```python
from build123d import *

# Parameters (mm, degrees)
SKETCH2_W               = 34
SKETCH2_H               = 40
BOSS_EXTRUDE1_DEPTH     = 3
SKETCH3_W               = 5
SKETCH3_H               = 40
BOSS_EXTRUDE2_DEPTH     = 37
CUT_EXTRUDE1_REACH      = 72.036
SKETCH4_R               = 1.35
SKETCH4_W               = 29
SKETCH4_H               = 28
SKETCH5_W               = 53
SKETCH5_H               = 40
BOSS_EXTRUDE3_DEPTH     = 5
SKETCH6_W               = 43
SKETCH6_H               = 30
BOSS_EXTRUDE4_DEPTH     = 36.85
SKETCH7_W               = 53
SKETCH7_H               = 40
BOSS_EXTRUDE5_DEPTH     = 5
SKETCH8_W               = 5
SKETCH8_H               = 40
BOSS_EXTRUDE6_DEPTH     = 40
SKETCH8_3_W             = 2
SKETCH8_3_H             = 40
BOSS_EXTRUDE7_DEPTH     = 5
CUT_EXTRUDE2_DEPTH      = 108.532192854
CUT_EXTRUDE2_DEPTH_BACK = 108.532192854
SKETCH9_R               = 1.35
SKETCH9_R_2             = 5


with BuildPart() as part:
    # Sketch2 → Boss-Extrude1 (new body)
    with BuildSketch(Plane(origin=(0, 0, 0), x_dir=(1, 0, 0), z_dir=(0, 1, 0))):
        with Locations((17, 20)):
            Rectangle(SKETCH2_W, SKETCH2_H)
    extrude(amount=BOSS_EXTRUDE1_DEPTH)

    # Sketch3 → Boss-Extrude2 (add)
    with BuildSketch(Plane(origin=(0, 0, 0), x_dir=(1, 0, 0), z_dir=(0, 1, 0))):
        with Locations((-2.5, 20)):
            Rectangle(SKETCH3_W, SKETCH3_H)
        with Locations((36.5, 20)):
            Rectangle(SKETCH3_W, SKETCH3_H)
    extrude(amount=BOSS_EXTRUDE2_DEPTH)

    # Cut-Extrude1: up to this face of the body (flat: up to its plane)
    cut_extrude1_end = Plane(part.part.faces().sort_by_distance((39, 18.5, -20))[0])
    # Sketch4 → Cut-Extrude1 (cut, up to the picked face)
    with BuildSketch(Plane.ZY.offset(5), mode=Mode.PRIVATE) as cut_extrude1_sk1:
        with Locations((-2.8, 33.1)):
            Circle(SKETCH4_R)
    cut_extrude1_tool1 = split(extrude(cut_extrude1_sk1.sketch, amount=-CUT_EXTRUDE1_REACH, mode=Mode.PRIVATE), bisect_by=cut_extrude1_end, keep=Keep.BOTH, mode=Mode.PRIVATE)
    # Sketch4 → Cut-Extrude1 (cut, up to the picked face)
    with BuildSketch(Plane.ZY.offset(5), mode=Mode.PRIVATE) as cut_extrude1_sk2:
        with Locations((-2.8, 11.1)):
            Circle(SKETCH4_R)
    cut_extrude1_tool2 = split(extrude(cut_extrude1_sk2.sketch, amount=-CUT_EXTRUDE1_REACH, mode=Mode.PRIVATE), bisect_by=cut_extrude1_end, keep=Keep.BOTH, mode=Mode.PRIVATE)
    # Sketch4 → Cut-Extrude1 (cut, up to the picked face)
    with BuildSketch(Plane.ZY.offset(5), mode=Mode.PRIVATE) as cut_extrude1_sk3:
        with Locations((-9.1, 5.8)):
            Circle(SKETCH4_R)
    cut_extrude1_tool3 = split(extrude(cut_extrude1_sk3.sketch, amount=-CUT_EXTRUDE1_REACH, mode=Mode.PRIVATE), bisect_by=cut_extrude1_end, keep=Keep.BOTH, mode=Mode.PRIVATE)
    # Sketch4 → Cut-Extrude1 (cut, up to the picked face)
    with BuildSketch(Plane.ZY.offset(5), mode=Mode.PRIVATE) as cut_extrude1_sk4:
        with Locations((-37.4, 11.1)):
            Circle(SKETCH4_R)
    cut_extrude1_tool4 = split(extrude(cut_extrude1_sk4.sketch, amount=-CUT_EXTRUDE1_REACH, mode=Mode.PRIVATE), bisect_by=cut_extrude1_end, keep=Keep.BOTH, mode=Mode.PRIVATE)
    # Sketch4 → Cut-Extrude1 (cut, up to the picked face)
    with BuildSketch(Plane.ZY.offset(5), mode=Mode.PRIVATE) as cut_extrude1_sk5:
        with Locations((-31.1, 5.8)):
            Circle(SKETCH4_R)
    cut_extrude1_tool5 = split(extrude(cut_extrude1_sk5.sketch, amount=-CUT_EXTRUDE1_REACH, mode=Mode.PRIVATE), bisect_by=cut_extrude1_end, keep=Keep.BOTH, mode=Mode.PRIVATE)
    # Sketch4 → Cut-Extrude1 (cut, up to the picked face)
    with BuildSketch(Plane.ZY.offset(5), mode=Mode.PRIVATE) as cut_extrude1_sk6:
        with Locations((-37.4, 33.1)):
            Circle(SKETCH4_R)
    cut_extrude1_tool6 = split(extrude(cut_extrude1_sk6.sketch, amount=-CUT_EXTRUDE1_REACH, mode=Mode.PRIVATE), bisect_by=cut_extrude1_end, keep=Keep.BOTH, mode=Mode.PRIVATE)
    # Sketch4 → Cut-Extrude1 (cut, up to the picked face)
    with BuildSketch(Plane.ZY.offset(5), mode=Mode.PRIVATE) as cut_extrude1_sk7:
        with Locations((-20, 23)):
            Rectangle(SKETCH4_W, SKETCH4_H)
    cut_extrude1_tool7 = split(extrude(cut_extrude1_sk7.sketch, amount=-CUT_EXTRUDE1_REACH, mode=Mode.PRIVATE), bisect_by=cut_extrude1_end, keep=Keep.BOTH, mode=Mode.PRIVATE)
    add(cut_extrude1_tool1.solids().sort_by(Axis((-5, 33.1, -2.8), (1, 0, 0)))[0], mode=Mode.SUBTRACT)
    add(cut_extrude1_tool2.solids().sort_by(Axis((-5, 11.1, -2.8), (1, 0, 0)))[0], mode=Mode.SUBTRACT)
    add(cut_extrude1_tool3.solids().sort_by(Axis((-5, 5.8, -9.1), (1, 0, 0)))[0], mode=Mode.SUBTRACT)
    add(cut_extrude1_tool4.solids().sort_by(Axis((-5, 11.1, -37.4), (1, 0, 0)))[0], mode=Mode.SUBTRACT)
    add(cut_extrude1_tool5.solids().sort_by(Axis((-5, 5.8, -31.1), (1, 0, 0)))[0], mode=Mode.SUBTRACT)
    add(cut_extrude1_tool6.solids().sort_by(Axis((-5, 33.1, -37.4), (1, 0, 0)))[0], mode=Mode.SUBTRACT)
    add(cut_extrude1_tool7.solids().sort_by(Axis((-5, 23, -20), (1, 0, 0)))[0], mode=Mode.SUBTRACT)

    # Sketch5 → Boss-Extrude3 (add)
    with BuildSketch(Plane(origin=(0, 0, 0), x_dir=(-1, 0, 0), z_dir=(0, -1, 0))):
        with Locations((-17, 20)):
            Rectangle(SKETCH5_W, SKETCH5_H)
    extrude(amount=BOSS_EXTRUDE3_DEPTH)

    # Sketch6 → Boss-Extrude4 (add)
    with BuildSketch(Plane.XZ.offset(5)):
        with Locations((17, -20)):
            Rectangle(SKETCH6_W, SKETCH6_H)
    extrude(amount=BOSS_EXTRUDE4_DEPTH)

    # Sketch7 → Boss-Extrude5 (add)
    with BuildSketch(Plane.XZ.offset(41.85)):
        with Locations((19, -22)):
            Rectangle(SKETCH7_W, SKETCH7_H)
    extrude(amount=BOSS_EXTRUDE5_DEPTH)

    # Sketch8 → Boss-Extrude6 (add)
    with BuildSketch(Plane.XZ.offset(46.85)):
        with Locations((-7, -22)):
            Rectangle(SKETCH8_W, SKETCH8_H)
        with Locations((45, -22)):
            Rectangle(SKETCH8_W, SKETCH8_H)
    extrude(amount=BOSS_EXTRUDE6_DEPTH)

    # Sketch8<3> → Boss-Extrude7 (add)
    with BuildSketch(Plane.XZ.offset(46.85)):
        with Locations((46.5, -22)):
            Rectangle(SKETCH8_3_W, SKETCH8_3_H)
        with Locations((-8.5, -22)):
            Rectangle(SKETCH8_3_W, SKETCH8_3_H)
    extrude(amount=-BOSS_EXTRUDE7_DEPTH)

    # Sketch9 → Cut-Extrude2 (cut, two sides: drawn at the far end of the back side and taken through both)
    with BuildSketch(Plane.ZY.offset(-CUT_EXTRUDE2_DEPTH_BACK)):
        with BuildLine():
            Line((-2, -86.85), (-12, -86.85))
            ThreePointArc((-12, -86.85), (-4.928932188, -83.921067812), (-2, -76.85))
            Line((-2, -76.85), (-2, -86.85))
        make_face()
        with BuildLine():
            ThreePointArc((-32, -86.85), (-39.071067812, -83.921067812), (-42, -76.85))
            Line((-42, -76.85), (-42, -86.85))
            Line((-42, -86.85), (-32, -86.85))
        make_face()
        with Locations(Location((-14.221825407, -77.128174593, 0), (0, 0, 180))):
            Circle(SKETCH9_R)
        with Locations(Location((-22, -80.35, 0), (0, 0, 180))):
            Circle(SKETCH9_R)
        with Locations(Location((-29.778174593, -77.128174593, 0), (0, 0, 180))):
            Circle(SKETCH9_R)
        with Locations(Location((-29.778174593, -61.571825407, 0), (0, 0, 180))):
            Circle(SKETCH9_R)
        with Locations(Location((-33, -69.35, 0), (0, 0, 180))):
            Circle(SKETCH9_R)
        with Locations(Location((-22, -69.35, 0), (0, 0, 180))):
            Circle(SKETCH9_R_2)
        with Locations(Location((-11, -69.35, 0), (0, 0, 180))):
            Circle(SKETCH9_R)
        with Locations(Location((-14.221825407, -61.571825407, 0), (0, 0, 180))):
            Circle(SKETCH9_R)
        with Locations(Location((-22, -58.35, 0), (0, 0, 180))):
            Circle(SKETCH9_R)
    extrude(amount=CUT_EXTRUDE2_DEPTH + CUT_EXTRUDE2_DEPTH_BACK, mode=Mode.SUBTRACT)


solid = part.part
```
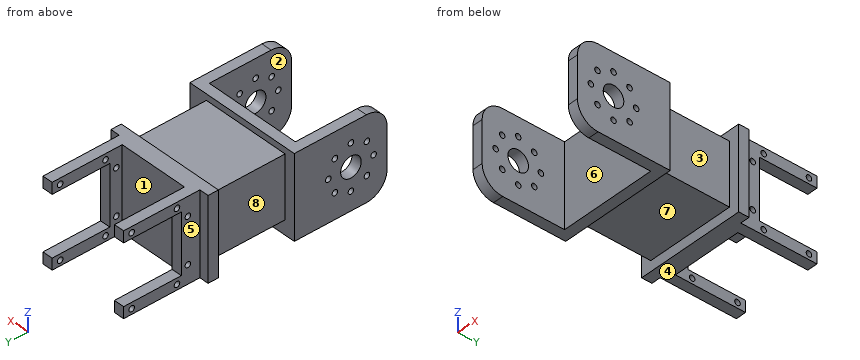
Design review of the part built by this model. Coordinates are the model's own, in mm. Face numbers are marked on the shaded views. A direction names the side the tool comes from. Coordinates: 2 decimals unless noted, no trailing zeros. Loops run counter-clockwise (first coordinate to the right, second up) from the corner with the lowest first, then second, coordinate; pieces in that order, holes last. Notation, with made-up numbers: (32.5, -23) - (39.5, -23) arc R27 ccw to (39.5, 9) - close; hole circle Ø11 at (54.5, -33). An arc over 180 degrees is marked (long way). Use CSV: the item, a comma, the result in double quotes. Start each with the question number.
1) Tool access review of the marked faces 1, 2, 3, 4 and 5: name each direction out of +Z, -Z, +X, -X, +Y, -Y from which nothing blocks a thin tool from reaching the whole face with its end or side.
2) Consider section C-C on x = 37. Write out the cut boundary in (y, z).
3) Consider section B-B on x = 17. Write out the cut boundary in (y, z), then the cut area to 3 significant figures.
4) Consider section D-D on y = -80.35. Write out the cut boundary in (x, z), then the cut area to 3 significant figures.
5) The part is to be moulded in two halves that separate along X. For the marked faces 6, 7 and 8, say which applies: +X half, -X half, draft (parallel to the pull), parting line (faces both ways), or undercut.
6) For pin 1 Ø1.6 at (y, z) = (33.1, -2.8) entering from -X; pin 2 Ø3 at (x, z) = (24, -34) entering from -Y; pin 3 Ø10 at (y, z) = (12.5, -30.5) entering from +X; pin 4 Ø2 at (x, y) = (29.5, -11.5) entering from -Z, all flat-tipped, find the tip position at first contact; note any pin that passes through.
7) Wall thickness on L1, parallel to Y at x = -3.2, z = -37.4; L2, parallel to X at y = -47, z = -10; L3, parallel to Y at x = 39.5, z = -9.5: over which ranges is each line inside the solid? List them lowest first. Write a range as from..to.
8) Consider section A-A on y = 5.8. Write out the cut boundary in (x, z), then the cut area to 3 significant figures.
Geometry says:
1,face 1,"+Z, -Z, +Y"
1,face 2,"+Z, -Z, -Y"
1,face 3,"+Z, -Z, +X"
1,face 4,"-Z, +X, -X, +Y"
1,face 5,"+Z, -Z, -X, +Y"
2,outline,"(-46.85, -42) - (-41.85, -42) - (-41.85, -35) - (-5, -35) - (-5, -40) - (37, -40) - (37, -34.5) - (9, -34.5) - (9, -5.5) - (37, -5.5) - (37, 0) - (-5, 0) - (-5, -5) - (-41.85, -5) - (-41.85, -2) - (-46.85, -2) - close; hole circle Ø2.7 at (5.8, -31.1); hole circle Ø2.7 at (5.8, -9.1); hole circle Ø2.7 at (11.1, -37.4); hole circle Ø2.7 at (11.1, -2.8); hole circle Ø2.7 at (33.1, -37.4); hole circle Ø2.7 at (33.1, -2.8)"
3,outline,"(-46.85, -42) - (-41.85, -42) - (-41.85, -35) - (-5, -35) - (-5, -40) - (3, -40) - (3, 0) - (-5, 0) - (-5, -5) - (-41.85, -5) - (-41.85, -2) - (-46.85, -2) - close"
3,area,"1,630 mm^2"
4,outline,"(-9.5, -41.37) - (-4.5, -41.37) - (-4.5, -23.35) - (-9.5, -23.35) - close; (-9.5, -20.65) - (-4.5, -20.65) - (-4.5, -2.63) - (-9.5, -2.63) - close; (42.5, -41.37) - (47.5, -41.37) - (47.5, -23.35) - (42.5, -23.35) - close; (42.5, -20.65) - (47.5, -20.65) - (47.5, -2.63) - (42.5, -2.63) - close"
4,area,"360 mm^2"
5,face 6,"undercut"
5,face 7,"draft"
5,face 8,"-X half"
6,pin 1,"through"
6,pin 2,"y = -46.85"
6,pin 3,"x = 39"
6,pin 4,"z = -35"
7,L1,"-46.85..-41.85, -5..9.75, 12.45..31.75, 34.45..37"
7,L2,"-9.5..-4.5, 42.5..47.5"
7,L3,"-46.85..-41.85, -5..0"
8,outline,"(-5, -40) - (0, -40) - (0, -32.45) - (-5, -32.45) - close; (-5, -29.75) - (0, -29.75) - (0, -10.45) - (-5, -10.45) - close; (-5, -7.75) - (0, -7.75) - (0, 0) - (-5, 0) - close; (34, -40) - (39, -40) - (39, -32.45) - (34, -32.45) - close; (34, -29.75) - (39, -29.75) - (39, -10.45) - (34, -10.45) - close; (34, -7.75) - (39, -7.75) - (39, 0) - (34, 0) - close"
8,area,"346 mm^2"
